Answer from the drawing. Dimensions are ordinates in mm from the lowest x, y and z of the part. Give positions to 0.01 mm unless a question says otherwise; leave off trailing zeros. Order: outer loops, then holes, each group sorted by start corner. A loop starts at its lowest first (then second) coordinate and runs counter-clockwise, first axis right, second up. Notation, with made-up numbers: (46, -36.5) - (104, -36.5) arc R27 ccw to (104, -11.5) - close; hole circle Ø9 at (25.25, 66). An arc over 180 degrees is marked (long way). One line per item, written item: value. Start each with the question number.
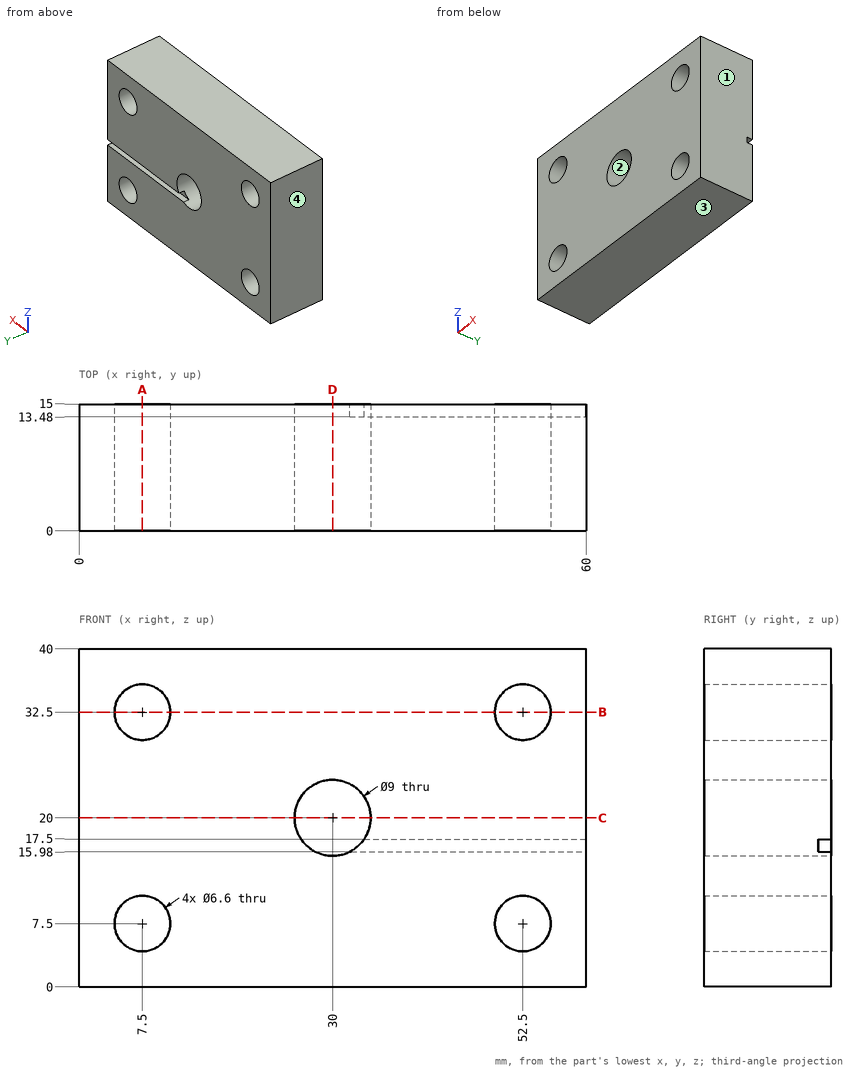
1) Section C-C on z = 20 is taken. Write down the section's boundary in (x, y).
2) This flat-tipped pin is pushed along its axis until it touches: pin 1 (0.8 mm diameter, centred on x = 47.5, z = 16.5, fed in from +Y). Where does it stop, or does it pass through?
3) Section D-D on x = 30 is taken. Write down the section's boundary in (y, z).
4) Section B-B on z = 32.5 is taken. Write down the section's boundary in (x, y), plus the area to 3 significant figures.
5) Section A-A on x = 7.5 is taken. Write down the section's boundary in (y, z), plus the area to 3 significant figures.
6) The mould has two halves that part along X. Classify the marked faces 1, 2, 3 and 4: +X half, -X half, draft (parallel to the pull), parting line (faces both ways), or undercut.
7) Find the intervals of material crossed by probe 1 along X at (y, z) = (7, 7.5); probe 2 along Z at (x, y) = (7.5, 11.5); probe 3 along X at (y, z) = (12.25, 31), in increasing order. Write a range as from..to.
Solved:
1. outline: (0, 0) - (25.5, 0) - (25.5, 15) - (0, 15) - close; (34.5, 0) - (60, 0) - (60, 15) - (34.5, 15) - close
2. pin 1: stops at y = 13.48
3. outline: (0, 0) - (15, 0) - (15, 15.5) - (0, 15.5) - close; (0, 24.5) - (15, 24.5) - (15, 40) - (0, 40) - close
4. outline: (0, 0) - (4.2, 0) - (4.2, 15) - (0, 15) - close; (10.8, 0) - (49.2, 0) - (49.2, 15) - (10.8, 15) - close; (55.8, 0) - (60, 0) - (60, 15) - (55.8, 15) - close
4. area: 702 mm2
5. outline: (0, 0) - (15, 0) - (15, 4.2) - (0, 4.2) - close; (0, 10.8) - (15, 10.8) - (15, 29.2) - (0, 29.2) - close; (0, 35.8) - (15, 35.8) - (15, 40) - (0, 40) - close
5. area: 402 mm2
6. face 1: +X half
6. face 2: undercut
6. face 3: draft
6. face 4: -X half
7. probe 1: x = 0..4.2, 10.8..49.2, 55.8..60
7. probe 2: z = 0..4.2, 10.8..29.2, 35.8..40
7. probe 3: x = 0..4.56, 10.44..49.56, 55.44..60
